Source: CAD feature listing. Evaluate the final solid. Frame: model axes, mm. Face numbers are marked on the shaded views. A direction names the side the tool comes from. Round coordinates to 2 decimals unless told otherwise and drop trailing zeros. Loops run counter-clockwise (first coordinate to the right, second up) from the corner with the lowest first, then second, coordinate; pieces in that order, holes last. Notation, with made-up numbers: (-29, 15) -> (-8, 15) arc R30 ccw to (-8, 49) -> close; hole circle Ø11 at (46, 35). An arc over 180 degrees is marked (long way). Put each result on its own line as item: value. Start each with the question number.
1. Cut plane B-B (y = 8.5). State how many separate pieces and enclosed holes the cut face has, then the cut area to 3 significant figures.
2. Draft query along X for the marked faces 4, 5 and 6. Return one class per face: pulls with the +X half, pulls with the -X half, needs draft (parallel to the pull), parting line crosses it, or undercut.
3. Cut plane C-C (z = -17). Return the cut outline in (x, y), then the cut area to 3 significant figures.
4. Material intervals for L1, parallel to Y at x = 5, z = -21; L2, parallel to Y at x = 25.5, z = -3; L3, parallel to Z at x = 90.5, y = 1.5, sorted ascending.
5. Cut plane A-A (x = 64.5). Return the cut outline in (y, z), then the cut area to 3 significant figures.
6. Contact query for flat-ended pins moving along their axis: pin 1 (3 mm diameter, centred on x = 32.5, z = -16.5, fed in from -Y); pin 2 (0.9 mm diameter, centred on x = 77, y = 7.5, fed in from -Z); pin 3 (1 mm diameter, centred on x = 53, z = -8, fed in from +Y); pin 4 (2 mm diameter, centred on x = 69, y = 6.5, fed in from +Z). Output: stop coordinate, or through.
7. Set-up query: the marked faces 1, 2 and 3. Return all of +Z, -Z, +X, -X, +Y, -Y with unobstructed straight access to the full face (end or side cutting, diameter ignored); none if empty.
```python
from build123d import *

# Parameters (mm, degrees)
SKETCH1_W            = 100
SKETCH1_H            = 16
BOSS_EXTRUDE1_DEPTH  = 3
SKETCH2_W            = 98
SKETCH2_H            = 14
CUT_EXTRUDE1_DEPTH   = 1
SKETCH5_W            = 20
SKETCH5_H            = 3
BOSS_EXTRUDE4_DEPTH  = 15
SKETCH6_W            = 20
SKETCH6_H            = 3
BOSS_EXTRUDE5_DEPTH  = 15
FILLET18_R           = 10
SKETCH7_W            = 3
SKETCH7_H            = 12
BOSS_EXTRUDE6_DEPTH  = 16
SKETCH8_W            = 6
SKETCH8_H            = 2
BOSS_EXTRUDE7_DEPTH  = 2
FILLET19_R           = 6
SKETCH10_W           = 60
SKETCH10_H           = 3
BOSS_EXTRUDE8_DEPTH  = 3
SKETCH11_W           = 60
SKETCH11_H           = 3
BOSS_EXTRUDE9_DEPTH  = 3
SKETCH12_W           = 0.95
SKETCH12_H           = 14
BOSS_EXTRUDE10_DEPTH = 3
SKETCH13_W           = 100
SKETCH13_H           = 0.95
BOSS_EXTRUDE11_DEPTH = 3
SKETCH14_W           = 0.95
SKETCH14_H           = 0.052088128
BOSS_EXTRUDE12_DEPTH = 3
SKETCH15_W           = 0.95
SKETCH15_H           = 0.047911872
SKETCH15_W_2         = 0.949734752
SKETCH15_H_2         = 0.052088128
BOSS_EXTRUDE13_DEPTH = 3


with BuildPart() as part:
    # Sketch1 → Boss-Extrude1 (new body)
    with BuildSketch(Plane(origin=(0, 0, 0), x_dir=(1, 0, 0), z_dir=(0, 1, 0))):
        with Locations((50, 8)):
            Rectangle(SKETCH1_W, SKETCH1_H)
    extrude(amount=BOSS_EXTRUDE1_DEPTH)

    # Sketch2 → Cut-Extrude1 (cut)
    with BuildSketch(Plane(origin=(0, 3, 0), x_dir=(1, 0, 0), z_dir=(0, 1, 0))):
        with Locations((50, 8)):
            Rectangle(SKETCH2_W, SKETCH2_H)
    extrude(amount=-CUT_EXTRUDE1_DEPTH, mode=Mode.SUBTRACT)

    # Sketch5 → Boss-Extrude4 (add)
    with BuildSketch(Plane.XY):
        with Locations((10, 1.5)):
            Rectangle(SKETCH5_W, SKETCH5_H)
        with Locations((90, 1.5)):
            Rectangle(SKETCH5_W, SKETCH5_H)
    extrude(amount=BOSS_EXTRUDE4_DEPTH)

    # Sketch6 → Boss-Extrude5 (add)
    with BuildSketch(Plane(origin=(0, 0, -16), x_dir=(-1, 0, 0), z_dir=(0, 0, -1))):
        with Locations((-90, 1.5)):
            Rectangle(SKETCH6_W, SKETCH6_H)
        with Locations((-10, 1.5)):
            Rectangle(SKETCH6_W, SKETCH6_H)
    extrude(amount=BOSS_EXTRUDE5_DEPTH)

    # Fillet18
    fillet18_edges = [part.edges().sort_by_distance(p)[0] for p in [
        (20, 1.5, 15),
        (0, 1.5, 15),
        (80, 1.5, 15),
        (100, 1.5, 15),
        (0, 1.5, -31),
        (20, 1.5, -31),
        (80, 1.5, -31),
        (100, 1.5, -31),
    ]]
    fillet(fillet18_edges, radius=FILLET18_R - 0.0001)  # a hair under: the kernel refuses the full size

    # Sketch7 → Boss-Extrude6 (add)
    with BuildSketch(Plane(origin=(0, 2, 0), x_dir=(1, 0, 0), z_dir=(0, 1, 0))):
        with Locations((95, 8)):
            Rectangle(SKETCH7_W, SKETCH7_H)
        with Locations((86, 8)):
            Rectangle(SKETCH7_W, SKETCH7_H)
        with Locations((77, 8)):
            Rectangle(SKETCH7_W, SKETCH7_H)
        with Locations((68, 8)):
            Rectangle(SKETCH7_W, SKETCH7_H)
        with Locations((59, 8)):
            Rectangle(SKETCH7_W, SKETCH7_H)
        with Locations((50, 8)):
            Rectangle(SKETCH7_W, SKETCH7_H)
        with Locations((41, 8)):
            Rectangle(SKETCH7_W, SKETCH7_H)
        with Locations((32, 8)):
            Rectangle(SKETCH7_W, SKETCH7_H)
        with Locations((23, 8)):
            Rectangle(SKETCH7_W, SKETCH7_H)
        with Locations((14, 8)):
            Rectangle(SKETCH7_W, SKETCH7_H)
        with Locations((5, 8)):
            Rectangle(SKETCH7_W, SKETCH7_H)
    extrude(amount=BOSS_EXTRUDE6_DEPTH)

    # Sketch8 → Boss-Extrude7 (add)
    with BuildSketch(Plane(origin=(0, 2, 0), x_dir=(1, 0, 0), z_dir=(0, 1, 0))):
        with Locations((90.5, 8)):
            Rectangle(SKETCH8_W, SKETCH8_H)
        with Locations((81.5, 8)):
            Rectangle(SKETCH8_W, SKETCH8_H)
        with Locations((72.5, 8)):
            Rectangle(SKETCH8_W, SKETCH8_H)
        with Locations((63.5, 8)):
            Rectangle(SKETCH8_W, SKETCH8_H)
        with Locations((54.5, 8)):
            Rectangle(SKETCH8_W, SKETCH8_H)
        with Locations((45.5, 8)):
            Rectangle(SKETCH8_W, SKETCH8_H)
        with Locations((36.5, 8)):
            Rectangle(SKETCH8_W, SKETCH8_H)
        with Locations((27.5, 8)):
            Rectangle(SKETCH8_W, SKETCH8_H)
        with Locations((18.5, 8)):
            Rectangle(SKETCH8_W, SKETCH8_H)
        with Locations((9.5, 8)):
            Rectangle(SKETCH8_W, SKETCH8_H)
    extrude(amount=BOSS_EXTRUDE7_DEPTH)

    # Fillet19
    fillet19_edges = [part.edges().sort_by_distance(p)[0] for p in [
        (95, 18, -2),
        (95, 18, -14),
        (86, 18, -2),
        (86, 18, -14),
        (77, 18, -2),
        (77, 18, -14),
        (68, 18, -2),
        (68, 18, -14),
        (59, 18, -2),
        (59, 18, -14),
        (50, 18, -2),
        (50, 18, -14),
        (41, 18, -2),
        (41, 18, -14),
        (32, 18, -2),
        (32, 18, -14),
        (23, 18, -14),
        (23, 18, -2),
        (14, 18, -2),
        (14, 18, -14),
        (5, 18, -2),
        (5, 18, -14),
    ]]
    fillet(fillet19_edges, radius=FILLET19_R - 0.0001)  # a hair under: the kernel refuses the full size

    # Sketch10 → Boss-Extrude8 (add)
    with BuildSketch(Plane(origin=(0, 0, -16), x_dir=(-1, 0, 0), z_dir=(0, 0, -1))):
        with Locations((-50, 1.5)):
            Rectangle(SKETCH10_W, SKETCH10_H)
    extrude(amount=BOSS_EXTRUDE8_DEPTH)

    # Sketch11 → Boss-Extrude9 (add)
    with BuildSketch(Plane.XY):
        with Locations((50, 1.5)):
            Rectangle(SKETCH11_W, SKETCH11_H)
    extrude(amount=BOSS_EXTRUDE9_DEPTH)

    # Sketch12 → Boss-Extrude10 (add)
    with BuildSketch(Plane(origin=(0, 3, 0), x_dir=(1, 0, 0), z_dir=(0, 1, 0))):
        with Locations((99.525, 7.997911872)):
            Rectangle(SKETCH12_W, SKETCH12_H)
        with Locations((0.475, 7.997911872)):
            Rectangle(SKETCH12_W, SKETCH12_H)
    extrude(amount=BOSS_EXTRUDE10_DEPTH)

    # Sketch13 → Boss-Extrude11 (add)
    with BuildSketch(Plane(origin=(0, 3, 0), x_dir=(1, 0, 0), z_dir=(0, 1, 0))):
        with Locations((50, 15.525)):
            Rectangle(SKETCH13_W, SKETCH13_H)
        with Locations((50, 0.475)):
            Rectangle(SKETCH13_W, SKETCH13_H)
    extrude(amount=BOSS_EXTRUDE11_DEPTH)

    # Sketch14 → Boss-Extrude12 (add)
    with BuildSketch(Plane(origin=(0, 3, 0), x_dir=(1, 0, 0), z_dir=(0, 1, 0))):
        with Locations((0.475, 15.023955936)):
            Rectangle(SKETCH14_W, SKETCH14_H)
    extrude(amount=BOSS_EXTRUDE12_DEPTH)

    # Sketch15 → Boss-Extrude13 (add)
    with BuildSketch(Plane(origin=(0, 3, 0), x_dir=(1, 0, 0), z_dir=(0, 1, 0))):
        with Locations((0.475, 0.973955936)):
            Rectangle(SKETCH15_W, SKETCH15_H)
        with Locations((99.525132624, 0.973955936)):
            Rectangle(SKETCH15_W_2, SKETCH15_H)
        with Locations((99.525, 15.023955936)):
            Rectangle(SKETCH15_W, SKETCH15_H_2)
    extrude(amount=BOSS_EXTRUDE13_DEPTH)


solid = part.part
```
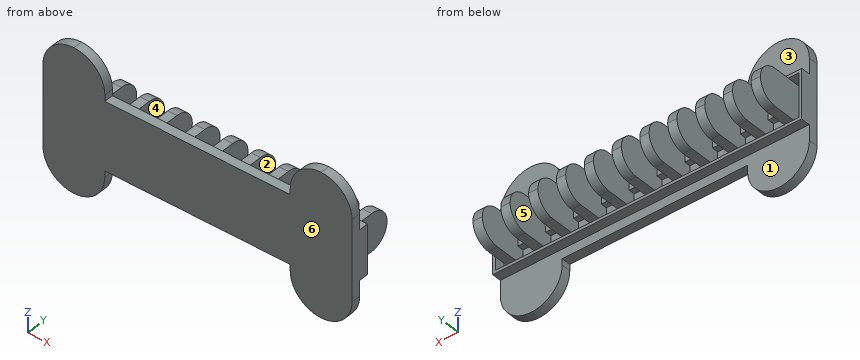
Solution:
1. separate pieces: 11
1. enclosed holes: 0
1. area: 396 mm^2
2. face 4: undercut
2. face 5: undercut
2. face 6: needs draft
3. outline: (0, 0) -> (100, 0) -> (100, 3) -> (0, 3) -> close
3. area: 300 mm^2
4. L1: y = 0 to 3
4. L2: y = 0 to 2
4. L3: z = -30.99 to 14.99
5. outline: (0, -19) -> (3, -19) -> (3, -16) -> (6, -16) -> (6, -15.05) -> (3, -15.05) -> (3, -15) -> (2, -15) -> (2, -9) -> (4, -9) -> (4, -7) -> (2, -7) -> (2, -1) -> (3, -1) -> (3, -0.95) -> (6, -0.95) -> (6, 0) -> (3, 0) -> (3, 3) -> (0, 3) -> close
5. area: 61.7 mm^2
6. pin 1: stops at y = 0
6. pin 2: stops at z = -14
6. pin 3: stops at y = 4
6. pin 4: stops at z = 0
7. face 1: -Z, +X, -X, +Y
7. face 2: +Y
7. face 3: +Z, +X, -X, +Y
